The listing builds one solid part. Answer for the finished solid, in the listing's coordinates (mm). A direction names the side the tool comes from. Round coordinates to 2 decimals unless told otherwise and drop trailing zeros. Loops run counter-clockwise (first coordinate to the right, second up) from the corner with the lowest first, then second, coordinate; pieces in that order, holes last. Notation, with made-up numbers: (-2, -0.75) - (15, -0.75) arc R25 ccw to (15, 28.25) - close; hole circle Ø4 at (-20, -2.5). An arc over 180 degrees is marked (long way). Write item = value, one per line. Start each with the question number.
1) Section B-B, the plane x = 41.5 is taken. Determine the outline of the cut face in (y, z).
2) Section C-C, the plane y = 8 is taken. Determine the outline of the cut face in (x, z).
3) Given pin 1 Ø8 at (y, z) = (23.5, 13.5) entering from -X; pin 2 Ø4.5 at (y, z) = (45.5, 6) entering from +X; pin 3 Ø7.5 at (x, z) = (7.5, 4) entering from +Y, each flat-ended and moving along its own axis, determine where each tip first touches the part or whether it passes through.
4) Section D-D, the plane x = 67.5 is taken. Determine the outline of the cut face in (y, z), and give its area (3 significant figures).
5) For a pull along Z with two mould halves and no side action, classify faces 5 (the cylindrical face through (76.179, 8.669, 10.903)), 6 (the flat face through (44, 28, 0)), 7 (the flat face through (44, 0, 8)) as released by +Z, released by -Z, zero draft, split by the parting line, or undercut.
6) Section A-A, the plane y = 50.8 is taken. Determine the outline of the cut face in (x, z).
7) A tool of negligible diameter and unlimited length cuts with its end or side. For faces 1 (the flat face through (77, 12.7, 2)), 2 (the flat face through (3, 4.75, 9)), 3 (the flat face through (15.748, 36, 8)), 4 (the flat face through (44, 28, 15.24)), from which of +Z, -Z, +X, -X, +Y, -Y can it reach the whole face along a straight path? Write none if from no direction.
8) Straight lines are drawn through the part: line 1 along Y through (x, z) = (76, 5.25); line 2 along X through (y, z) = (28, 14); line 3 along X through (y, z) = (9, 11). For each, find the intervals that lie inside material, in ascending order.
Autodesk Inventor part; units mm, degrees
ref_plane "YZ Plane" through (0, 0, 0) normal (1, 0, 0) x (0, 1, 0)
ref_plane "XZ Plane" through (0, 0, 0) normal (0, 1, 0) x (-1, 0, 0)
ref_plane "XY Plane" through (0, 0, 0) normal (0, 0, 1) x (1, 0, 0)
sketch "Sketch1" plane through (0, 0, 0) normal (0, 0, 1) x (1, 0, 0)
  line L0 (0, 0) -> (88.9, 0)
  line L1 (88.9, 0) -> (88.9, 12.7)
  line L2 (0, 12.7) -> (0, 0)
  line L3 (0, 12.7) -> (0, 0)
  circle A0 centre (37.338, 50.8) radius 14.2875
  line L4 (0, 0) -> (0, 12.7)
  line L5 (0, 0) -> (0, 12.7)
  line L6 (0, 12.7) -> (15.748, 12.7)
  line L7 (13.208, 0) -> (0, 0)
  line L8 (15.748, 12.7) -> (0, 12.7)
  line L9 (15.748, 54.61) -> (15.748, 12.7)
  line L10 (88.9, 0) -> (62.992, 0)
  line L11 (73.152, 12.7) -> (88.9, 12.7)
  line L12 (88.9, 12.7) -> (88.9, 0)
  line L13 (73.152, 12.7) -> (73.152, 54.61)
  line L14 (60.452, 71.222) -> (28.448, 71.222)
  line L15 (15.748, 54.61) -> (15.748, 58.522)
  line L16 (73.152, 58.522) -> (73.152, 54.61)
  arc A1 (28.448, 71.222) -> (15.748, 58.522) centre (28.448, 58.522) ccw
  arc A2 (73.152, 58.522) -> (60.452, 71.222) centre (60.452, 58.522) ccw
  point P0 (65.9232, 76.2)
  point P1 (0, 12.7)
  dimension "d9" = 28.575
  dimension "d10" = 88.9
  dimension "d56" = 12.7
  dimension "d57" = 15.748
  dimension "d79" = 21.59
  dimension "d83" = 15.748
  dimension "d87" = 12.7
  dimension "d111" = 41.91
  dimension "d112" = 41.91
  dimension "d118" = 25.4
  dimension "d119" = 12.7
extrude "Extrusion7" add sketch "Sketch1" along normal blind 15.24
sketch "Sketch9" plane through (73.152, 12.7, 0) normal (0, 1, 0) x (1, 0, 0)
  point P0 (-73.152, 0)
  point P1 (8.0463, -7.7031)
hole "Hole4" at (81.1983, 12.7, 7.7031) direction (0, -1, 0) diameter 8.4328 end through all counterbore diameter 11.9062 counterbore depth 7.9502
sketch "Sketch10" plane through (0.0713, 12.7, -0.0767) normal (0, 1, 0) x (1, 0, 0)
  point P0 (-75.692, 0)
  point P1 (7.4278, -7.7745)
hole "Hole5" at (7.4991, 12.7, 7.6977) direction (0, -1, 0) diameter 8.4328 end through all counterbore diameter 11.9062 counterbore depth 7.9502
properties part number "Updated Support"
Geometry check:
q1.outline = (0, 0) - (37.13, 0) - (37.13, 15.24) - (0, 15.24) - close; (64.47, 0) - (71.22, 0) - (71.22, 15.24) - (64.47, 15.24) - close
q2.outline = (0, 0) - (88.9, 0) - (88.9, 15.24) - (0, 15.24) - close; hole circle Ø11.91 at (7.5, 7.7); hole circle Ø11.91 at (81.2, 7.7)
q3.pin_1 = 15.75
q3.pin_2 = 73.15
q3.pin_3 = 12.7
q4.outline = (0, 0) - (69.09, 0) - (69.09, 15.24) - (0, 15.24) - close
q4.area = 1,050 mm2
q5.face_5 = undercut
q5.face_6 = released by -Z
q5.face_7 = zero draft
q6.outline = (15.75, 0) - (23.05, 0) - (23.05, 15.24) - (15.75, 15.24) - close; (51.63, 0) - (73.15, 0) - (73.15, 15.24) - (51.63, 15.24) - close
q7.face_1 = +Z, -Z, +X, +Y
q7.face_2 = +Y
q7.face_3 = +Z, -Z, -X, +Y
q7.face_4 = +Z, +X, -X, +Y, -Y
q8.line_1 = 0 to 4.75
q8.line_2 = 15.75 to 73.15
q8.line_3 = 0 to 2.55, 12.45 to 76.24, 86.16 to 88.9
